Autodesk Inventor part; units mm, degrees
ref_plane "YZ Plane" through (0, 0, 0) normal (1, 0, 0) x (0, 1, 0)
ref_plane "XZ Plane" through (0, 0, 0) normal (0, 1, 0) x (-1, 0, 0)
ref_plane "XY Plane" through (0, 0, 0) normal (0, 0, 1) x (1, 0, 0)
sketch "Sketch1" plane through (0, 0, 0) normal (0, 0, 1) x (1, 0, 0)
  line L0 (18.6512, 0) -> (-18.6512, 0) construction
  line L1 (-27.5858, -4.4915) -> (0, 32.6237)
  line L2 (0, 32.6237) -> (27.5858, -4.4915)
  line L3 (27.5858, -4.4915) -> (-27.5858, -4.4915)
  line L4 (0, 32.6237) -> (0, 9.3762) construction
  line L5 (0, 9.3762) -> (-27.5858, -4.4915) construction
  line L6 (0, 9.3762) -> (27.5858, -4.4915) construction
  point P0 (0, 0)
  point P1 (0, 22.6237)
  point P2 (0, 0)
  dimension "d0" = 37.3025
  dimension "d1" = 22.6237
  dimension "d2" = 10
  dimension "d3" = 10
  dimension "d21" = 26.689
  dimension "d22" = 26.689
extrude "Extrusion1" add sketch "Sketch1" along normal blind 3
hole "Hole1" at (0, 22.6237, 0) at (18.6512, 0, 0) at (-18.6512, 0, 0) direction (0, 0, 1) diameter 3.4 depth 7 tip angle 118 countersink diameter 6.3 countersink angle 90
hole "Hole2" at (0, 9.3762, 0) direction (0, 0, 1) diameter 4.5 depth 7 tip angle 118
fillet "Fillet1" radius 5 3 edges at (0, 32.6237, 1.5) (27.5858, -4.4915, 1.5) (-27.5858, -4.4915, 1.5)
equation "\"d21\" = d22"
properties part number "Idle Ball Mount"
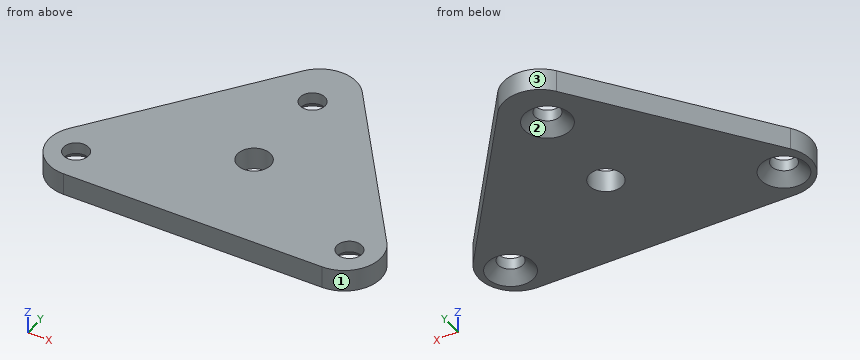
Geometry check sheet. Reference: the model listing, model coordinates, mm. Face numbers are marked on the shaded views. Give positions to 0.01 mm unless a question says otherwise; leave off trailing zeros. Write each loop counter-clockwise with the first axis right and the second up, starting at its lowest first coordinate (ties: lowest second). Pieces come first, ordered by that corner, then holes.
1) Cross-section at C-C (y = 8). Record the boundary of the cut face in (x, z), plus the area to 3 significant figures.
Values follow:
outline: (-18.3, 0) - (-1.78, 0) - (-1.78, 3) - (-18.3, 3) - close; (1.78, 0) - (18.3, 0) - (18.3, 3) - (1.78, 3) - close
area: 99.1 mm2
2) Cross-section at A-A (x = 0). Record the boundary of the cut face in (y, z), plus the area to 3 significant figures.
Values follow:
outline: (-4.49, 0) - (7.13, 0) - (7.13, 3) - (-4.49, 3) - close; (11.63, 0) - (19.47, 0) - (20.92, 1.45) - (20.92, 3) - (11.63, 3) - close; (24.32, 1.45) - (25.77, 0) - (29.24, 0) - (29.24, 3) - (24.32, 3) - close
area: 75.4 mm2
3) Cross-section at D-D (y = 0). Record the boundary of the cut face in (x, z), plus the area to 3 significant figures.
Values follow:
outline: (-22.61, 0) - (-21.8, 0) - (-20.35, 1.45) - (-20.35, 3) - (-22.61, 3) - close; (-16.95, 1.45) - (-15.5, 0) - (15.5, 0) - (16.95, 1.45) - (16.95, 3) - (-16.95, 3) - close; (20.35, 1.45) - (21.8, 0) - (22.61, 0) - (22.61, 3) - (20.35, 3) - close
area: 111 mm2
4) Go/stop test with flat-tipped pins: pin 1 Ø4 at (x, y) = (0, 9.38) entering from +Z; pin 2 Ø2 at (x, y) = (7, 21) entering from -Z; pin 3 Ø4.5 at (x, y) = (-18.65, 0) entering from -Z; pin 4 Ø4 at (x, y) = (18.65, 0) entering from -Z. Record where each tip stops, or that it passes through.
Values follow:
pin 1: passes through
pin 2: stops at z = 0
pin 3: stops at z = 0.9
pin 4: stops at z = 1.15
5) Cross-section at B-B (z = 0.6). Record the boundary of the cut face in (x, y).
Values follow:
outline: (-21.65, 3.49) arc R5 ccw to (-17.64, -4.49) - (17.64, -4.49) arc R5 ccw to (21.65, 3.49) - (4.01, 27.22) arc R5 ccw to (-4.01, 27.22) - close; hole circle Ø5.1 at (-18.65, 0); hole circle Ø5.1 at (0, 22.62); hole circle Ø4.5 at (0, 9.38); hole circle Ø5.1 at (18.65, 0)
6) Thickness scan on line 1 (Y direction, x = 0, z = 2.25); line 2 (X direction, y = 0, z = 2.6); line 3 (Y direction, x = 0, z = 1.4). Record the ranges inside material, lowest first.
Values follow:
line 1: y = -4.49 to 7.13, 11.63 to 20.92, 24.32 to 29.24
line 2: x = -22.61 to -20.35, -16.95 to 16.95, 20.35 to 22.61
line 3: y = -4.49 to 7.13, 11.63 to 20.87, 24.37 to 29.24
7) Release check for a two-part mould opening along X. For the marked faces 1, 2 and 3 record: released by +X, released by -X, zero draft, split by the parting line, or undercut.
Values follow:
face 1: released by +X
face 2: undercut
face 3: split by the parting line
